```python
from build123d import *

# Parameters (mm, degrees)
SKETCH1_R           = 13
SKETCH1_R_2         = 3
BOSS_EXTRUDE1_DEPTH = 6
CIRPATTERN1_DEPTH   = 6


# Read off the part's stored shape, not the designer's step: CirPattern1
with BuildPart() as part:
    # Sketch1 → Boss-Extrude1 (new body)
    with BuildSketch(Plane(origin=(0, 0, 0), x_dir=(1, 0, 0), z_dir=(0, 1, 0))):
        with Locations(Location((0, 0, 0), (0, 0, 270))):
            Circle(SKETCH1_R)
        with Locations(Location((0, 0, 0), (0, 0, 270))):
            Circle(SKETCH1_R_2, mode=Mode.SUBTRACT)
        with BuildLine():
            ThreePointArc((-3.111111111, 6.270644915), (-1.597730514, 6.815222462), (0, 7))
            ThreePointArc((0, 7), (1.597730514, 6.815222462), (3.111111111, 6.270644915))
            ThreePointArc((3.111111111, 6.270644915), (4.451361972, 6.722006887), (4, 8.062257748))
            ThreePointArc((4, 8.062257748), (2.054224947, 8.762428879), (0, 9))
            ThreePointArc((0, 9), (-2.054224947, 8.762428879), (-4, 8.062257748))
            ThreePointArc((-4, 8.062257748), (-4.451361972, 6.722006887), (-3.111111111, 6.270644915))
        make_face(mode=Mode.SUBTRACT)
    extrude(amount=BOSS_EXTRUDE1_DEPTH)

    # CirPattern1 outline → CirPattern1 (cut)
    with BuildSketch(Plane(origin=(0, 0, 0), x_dir=(1, 0, 0), z_dir=(0, 1, 0))):
        with BuildLine():
            ThreePointArc((8.062257748, 4), (6.722006887, 4.451361972), (6.270644915, 3.111111111))
            ThreePointArc((6.270644915, 3.111111111), (7, 0), (6.270644915, -3.111111111))
            ThreePointArc((6.270644915, -3.111111111), (6.722006887, -4.451361972), (8.062257748, -4))
            ThreePointArc((8.062257748, -4), (9, 0), (8.062257748, 4))
        make_face()
        with BuildLine():
            ThreePointArc((4, -8.062257748), (4.451361972, -6.722006887), (3.111111111, -6.270644915))
            ThreePointArc((3.111111111, -6.270644915), (0, -7), (-3.111111111, -6.270644915))
            ThreePointArc((-3.111111111, -6.270644915), (-4.451361972, -6.722006887), (-4, -8.062257748))
            ThreePointArc((-4, -8.062257748), (0, -9), (4, -8.062257748))
        make_face()
        with BuildLine():
            ThreePointArc((-8.062257748, -4), (-6.722006887, -4.451361972), (-6.270644915, -3.111111111))
            ThreePointArc((-6.270644915, -3.111111111), (-7, 0), (-6.270644915, 3.111111111))
            ThreePointArc((-6.270644915, 3.111111111), (-6.722006887, 4.451361972), (-8.062257748, 4))
            ThreePointArc((-8.062257748, 4), (-9, 0), (-8.062257748, -4))
        make_face()
    extrude(amount=CIRPATTERN1_DEPTH, mode=Mode.SUBTRACT)


solid = part.part
```
Part model, mm, in its own coordinate system. A direction names the side the tool comes from. Give positions to 0.01 mm unless a question says otherwise; leave off trailing zeros. Order: outer loops, then holes, each group sorted by start corner. A loop starts at its lowest first (then second) coordinate and runs counter-clockwise, first axis right, second up. Notation, with made-up numbers: (51, 85.5) - (58, 85.5) arc R18 cw to (58, 95.5) - close; hole circle Ø10 at (89.5, 42). An arc over 180 degrees is marked (long way). Use one line per item in the form item = value.
Item 1: Which spindle directions (+Z, -Z, +X, -X, +Y, -Y) get a long thin tool onto all of the face, cutting with end or side? Do faces 1 (the face through (-9, 3, 0)), 2 (the face through (-3, 0, 3)). Say none if no direction does.
Solution:
face_1 = +Y, -Y
face_2 = +Z, -Z, +X, -X, -Y
Item 2: Slice it at D-D on z = 5. Give the cut face in (x, y), and give its area (3 significant figures).
Solution:
outline = (-12, 0) - (12, 0) - (12, 6) - (-12, 6) - close
area = 144 mm2
Item 3: Probe probe 1 along X at (y, z) = (3.05, 0); probe 2 along Z at (x, y) = (3.5, 1.3); probe 3 along X at (y, z) = (1.65, -1.25). List the from-to ranges inside material, lowest first. Write a range as from..to.
Solution:
probe_1 = -13..-9, -7..-3, 3..7, 9..13
probe_2 = -12.52..-8.29, -6.17..6.17, 8.29..12.52
probe_3 = -12.94..-8.91, -6.89..-2.73, 2.73..6.89, 8.91..12.94
Item 4: Two-plate mould, pull along X, no slides. Class faces 3 (the face through (-6.7, 2.96, -4.44)), 4 (the face through (-7.91, 2.958, -10.316)), 5 (the face through (9, 3, 0)), 6 (the face through (-3, 6, 3)): released by +X, released by -X, zero draft, split by the parting line, or undercut.
Solution:
face_3 = undercut
face_4 = split by the parting line
face_5 = undercut
face_6 = zero draft
Item 5: Slice it at A-A on y = 4.75. Give the cut face in (x, z).
Solution:
outline = circle Ø26 at (0, 0); hole (-8.06, -4) arc R1 ccw to (-6.27, -3.11) arc R7 cw to (-6.27, 3.11) arc R1 ccw to (-8.06, 4) arc R9 ccw to start; hole (-4, -8.06) arc R9 ccw to (4, -8.06) arc R1 ccw to (3.11, -6.27) arc R7 cw to (-3.11, -6.27) arc R1 ccw to start; hole (-4, 8.06) arc R1 ccw to (-3.11, 6.27) arc R7 cw to (3.11, 6.27) arc R1 ccw to (4, 8.06) arc R9 ccw to start; hole circle Ø6 at (0, 0); hole (6.27, -3.11) arc R1 ccw to (8.06, -4) arc R9 ccw to (8.06, 4) arc R1 ccw to (6.27, 3.11) arc R7 cw to start
Item 6: Pin check, flat tips, straight feed: pin 1 Ø1 at (y, z) = (2, -3) entering from -X; pin 2 Ø1.5 at (y, z) = (5, 4) entering from +X. Stop position of each tip, or through.
Solution:
pin_1 = -12.76
pin_2 = 12.59
Item 7: Slice it at B-B on x = 2. Give the cut face in (y, z), and give its area (3 significant figures).
Solution:
outline = (0, -12.85) - (6, -12.85) - (6, -8.77) - (0, -8.77) - close; (0, -6.71) - (6, -6.71) - (6, -2.24) - (0, -2.24) - close; (0, 2.24) - (6, 2.24) - (6, 6.71) - (0, 6.71) - close; (0, 8.77) - (6, 8.77) - (6, 12.85) - (0, 12.85) - close
area = 103 mm2
Item 8: Slice it at C-C on z = 0. Give the cut face in (x, y).
Solution:
outline = (-13, 0) - (-9, 0) - (-9, 6) - (-13, 6) - close; (-7, 0) - (-3, 0) - (-3, 6) - (-7, 6) - close; (3, 0) - (7, 0) - (7, 6) - (3, 6) - close; (9, 0) - (13, 0) - (13, 6) - (9, 6) - close
